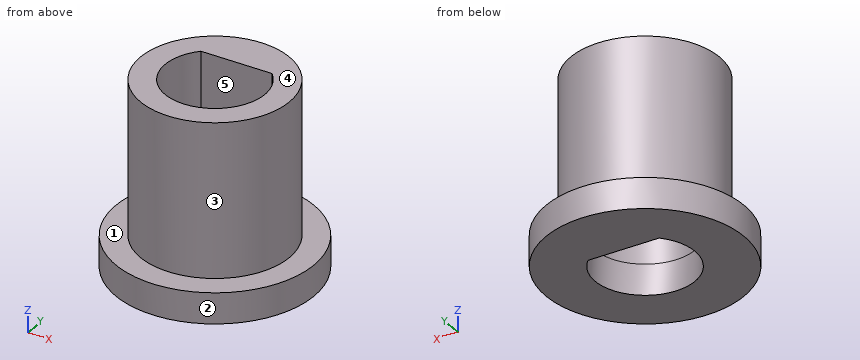
from build123d import *

# Parameters (mm, degrees)
SKETCH1_R           = 2.425
BOSS_EXTRUDE1_DEPTH = 5
BOSS_EXTRUDE2_START = -1
SKETCH1_4_R         = 3.225
SKETCH1_4_R_2       = 2.425
SKETCH1_4_R_3       = 1.625
BOSS_EXTRUDE2_DEPTH = 1


with BuildPart() as part:
    # Sketch1 → Boss-Extrude1 (new body)
    with BuildSketch(Plane.XY):
        Circle(SKETCH1_R)
        with BuildLine():
            Line((-1.17260394, 1.125), (1.17260394, 1.125))
            ThreePointArc((1.17260394, 1.125), (0, -1.625), (-1.17260394, 1.125))
        make_face(mode=Mode.SUBTRACT)
    extrude(amount=BOSS_EXTRUDE1_DEPTH)

    # Sketch1_4 → Boss-Extrude2 (add)
    # profile 1 of 3: a face of its own
    with BuildSketch(Plane.XY.offset(BOSS_EXTRUDE2_START)):
        Circle(SKETCH1_4_R)
        Circle(SKETCH1_4_R_2, mode=Mode.SUBTRACT)
    # profile 2 of 3: a face of its own
    with BuildSketch(Plane.XY.offset(BOSS_EXTRUDE2_START)):
        Circle(SKETCH1_4_R_2)
        Circle(SKETCH1_4_R_3, mode=Mode.SUBTRACT)
    # profile 3 of 3: a face of its own
    with BuildSketch(Plane.XY.offset(BOSS_EXTRUDE2_START)):
        with BuildLine():
            ThreePointArc((1.17260394, 1.125), (0, 1.625), (-1.17260394, 1.125))
            Line((-1.17260394, 1.125), (1.17260394, 1.125))
        make_face()
    extrude(amount=BOSS_EXTRUDE2_DEPTH)


solid = part.part
Could you check a few things on this model? Use its own coordinates, in mm. Face numbers are marked on the shaded views. A direction names the side the tool comes from. Give positions to 0.01 mm unless a question says otherwise; leave off trailing zeros. Order: outer loops, then holes, each group sorted by start corner. A loop starts at its lowest first (then second) coordinate and runs counter-clockwise, first axis right, second up. Notation, with made-up numbers: (76, -27.75) - (86, -27.75) arc R22 ccw to (86, -12.75) - close; hole circle Ø9 at (82, 28.25). An arc over 180 degrees is marked (long way). One line per question, with ' | ' between items. Start each with the question number.
Item 1: For the marked faces 1 and 2, which set-ups out of +Z, -Z, +X, -X, +Y, -Y let a thin tool reach every point of the face, with its end or its side?
Item 2: Thinking about a two-plate mould opening in Y: for the marked faces 3, 4 and 5, which applies, pulls with the +Y half, pulls with the -Y half, needs draft (parallel to the pull), parting line crosses it, or undercut?
Item 3: I'm going to push flat-ended pins straight in: pin 1 Ø3 at (x, z) = (2.5, 0) entering from +Y; pin 2 Ø1.2 at (x, z) = (0, 3) entering from -Y (3 decimals); pin 3 Ø3.5 at (x, y) = (0, 0) entering from -Z; pin 4 Ø1 at (x, z) = (1.5, 4) entering from -Y. Where does each tip first touch, or does it pass through?
Item 4: I want a section at D-D on x = 1.75. Write out the boundary of the cut face in (y, z), then the cut area to 3 significant figures.
Item 5: I want a section at A-A on x = 0. Write out the boundary of the cut face in (y, z) (3 decimals), then the cut area to 3 significant figures.
Item 6: I want a section at B-B on y = 0. Write out the boundary of the cut face in (x, z) (3 decimals), then the cut area to 3 significant figures.
Item 7: I want a section at C-C on z = 1.75. Write out the boundary of the cut face in (x, y) (3 decimals).
Item 8: I need wall thicknesses on probe 1 along Y at (x, z) = (0, 2.5) (3 decimals); probe 2 along Y at (x, z) = (0, -0.4) (3 decimals); probe 3 along Z at (x, y) = (-2.75, -0.5). Which ranges of each line are inside material? Lowest first, please. Write a range as [from, to].
Verdict:
1) face 1: +Z | face 2: +Z, -Z
2) face 3: parting line crosses it | face 4: needs draft | face 5: undercut
3) pin 1: y = 3.07 | pin 2: y = -2.425 | pin 3: z = -1 | pin 4: y = -2.21
4) outline: (-2.71, -1) - (2.71, -1) - (2.71, 0) - (1.68, 0) - (1.68, 5) - (-1.68, 5) - (-1.68, 0) - (-2.71, 0) - close | area: 22.2 mm^2
5) outline: (-3.225, -1) - (-1.625, -1) - (-1.625, 5) - (-2.425, 5) - (-2.425, 0) - (-3.225, 0) - close; (1.125, -1) - (3.225, -1) - (3.225, 0) - (2.425, 0) - (2.425, 5) - (1.125, 5) - close | area: 14.2 mm^2
6) outline: (-3.225, -1) - (-1.625, -1) - (-1.625, 5) - (-2.425, 5) - (-2.425, 0) - (-3.225, 0) - close; (1.625, -1) - (3.225, -1) - (3.225, 0) - (2.425, 0) - (2.425, 5) - (1.625, 5) - close | area: 11.2 mm^2
7) outline: circle Ø4.85 at (0, 0); hole (-1.173, 1.125) arc R1.625 ccw (long way) to (1.173, 1.125) - close
8) probe 1: [-2.425, -1.625], [1.125, 2.425] | probe 2: [-3.225, -1.625], [1.125, 3.225] | probe 3: [-1, 0]
